from build123d import *

# Parameters (mm, degrees)
SKETCH1_W           = 20
SKETCH1_H           = 20
BOSS_EXTRUDE1_DEPTH = 6
BOSS_EXTRUDE2_DEPTH = 26
SKETCH5_R           = 2
CUT_EXTRUDE1_DEPTH  = 32.176914536
CIRPATTERN1_COUNT   = 2
CIRPATTERN1_ANGLE   = 90
BOSS_EXTRUDE3_DEPTH = 20
SKETCH6_R           = 2
CUT_EXTRUDE2_DEPTH  = 38.416573868
CIRPATTERN2_COUNT   = 2
CIRPATTERN2_ANGLE   = 90
FILLET1_R           = 1


with BuildPart() as part:
    # Sketch1 → Boss-Extrude1 (new body)
    with BuildSketch(Plane(origin=(0, 0, 0), x_dir=(1, 0, 0), z_dir=(0, 1, 0))):
        Rectangle(SKETCH1_W, SKETCH1_H)
    extrude(amount=BOSS_EXTRUDE1_DEPTH)

    # Sketch2 → Boss-Extrude2 (add)
    with BuildSketch(Plane(origin=(0, 0, 0), x_dir=(1, 0, 0), z_dir=(0, 1, 0))):
        Polygon((-3, 10), (3, 10), (3, 8.1), (5.3, 8.1), (5.3, 6.48), (2.8, 4), (-2.8, 4), (-5.3, 6.48), (-5.3, 8.1), (-3, 8.1), align=None)
    boss_extrude2 = extrude(amount=BOSS_EXTRUDE2_DEPTH)

    # Sketch5 → Cut-Extrude1 (cut, through all)
    with BuildSketch(Plane.XY.offset(-4)):
        with Locations((0, 18)):
            Circle(SKETCH5_R)
    cut_extrude1 = extrude(amount=-CUT_EXTRUDE1_DEPTH, mode=Mode.SUBTRACT)

    # CirPattern1: Boss-Extrude2, Cut-Extrude1 ×2 about axis
    cirpattern1_axis = Axis((0, 0, 0), (0, 1, 0))
    add([boss_extrude2.rotate(cirpattern1_axis, i * CIRPATTERN1_ANGLE / (CIRPATTERN1_COUNT - 1)) for i in range(1, CIRPATTERN1_COUNT)])
    add([cut_extrude1.rotate(cirpattern1_axis, i * CIRPATTERN1_ANGLE / (CIRPATTERN1_COUNT - 1)) for i in range(1, CIRPATTERN1_COUNT)], mode=Mode.SUBTRACT)

    # Sketch4 → Boss-Extrude3 (add)
    with BuildSketch(Plane(origin=(10, 6.045130441, 0.430052004), x_dir=(0, 0, 1), z_dir=(1, 0, 0))):
        Polygon((-3.430052004, 6.045130441), (2.569947996, 6.045130441), (2.569947996, 4.145130441), (4.869947996, 4.145130441), (4.869947996, 2.525130441), (2.369947996, 0.045130441), (-3.230052004, 0.045130441), (-5.730052004, 2.525130441), (-5.730052004, 4.145130441), (-3.430052004, 4.145130441), align=None)
    boss_extrude3 = extrude(amount=BOSS_EXTRUDE3_DEPTH)

    # Sketch6 → Cut-Extrude2 (cut, through all)
    with BuildSketch(Plane(origin=(0, 6, 0), x_dir=(1, 0, 0), z_dir=(0, 1, 0))):
        with Locations(Location((22, 0, 0), (0, 0, 270))):
            Circle(SKETCH6_R)
    cut_extrude2 = extrude(amount=-CUT_EXTRUDE2_DEPTH, mode=Mode.SUBTRACT)

    # CirPattern2: Boss-Extrude3, Cut-Extrude2 ×2 about axis
    cirpattern2_axis = Axis((0, 0, 0), (0, -1, 0))
    add([boss_extrude3.rotate(cirpattern2_axis, i * CIRPATTERN2_ANGLE / (CIRPATTERN2_COUNT - 1)) for i in range(1, CIRPATTERN2_COUNT)])
    add([cut_extrude2.rotate(cirpattern2_axis, i * CIRPATTERN2_ANGLE / (CIRPATTERN2_COUNT - 1)) for i in range(1, CIRPATTERN2_COUNT)], mode=Mode.SUBTRACT)

    # Fillet1
    fillet1_edges = [part.edges().sort_by_distance(p)[0] for p in [
        (-10, 0, 0),
        (0, 0, -10),
        (10, 3, -10),
        (10, 3, 10),
        (-10, 3, 10),
        (-10, 3, -10),
    ]]
    fillet(fillet1_edges, radius=FILLET1_R)


solid = part.part
Can you work these out from the model? Positions are in its coordinate system, mm. A direction names the side the tool comes from. Give positions to 0.01 mm unless a question says otherwise; leave off trailing zeros. Order: outer loops, then holes, each group sorted by start corner. A loop starts at its lowest first (then second) coordinate and runs counter-clockwise, first axis right, second up. Notation, with made-up numbers: M -28.75,-34 L 0.25,-34 A16 cw 0.25,-25 Z; hole C 43.25,7 d6. An arc over 180 degrees is marked long. One line per item, written item: value.
Item 1: If we section it at D-D on x = 0: Write out the boundary of the cut face in (y, z), and give its area (3 significant figures).
Verdict:
outline: M 0,-9 A1 ccw 1,-10 L 16,-10 L 16,-4 L 6,-4 L 6,20 L 0,20 Z; M 0,24 L 6,24 L 6,30 L 0,30 Z; M 20,-10 L 26,-10 L 26,-4 L 20,-4 Z
area: 312 mm2
Item 2: If we section it at B-B on x = 22: Write out the boundary of the cut face in (y, z), and give its area (3 significant figures).
Verdict:
outline: M 0,-3 L 1.9,-3 L 1.9,-5.3 L 3.52,-5.3 L 6,-2.8 L 6,-2 L 0,-2 Z; M 0,2 L 6,2 L 6,2.8 L 3.52,5.3 L 1.9,5.3 L 1.9,3 L 0,3 Z
area: 24.7 mm2
Item 3: For pin 1 (0.6 mm diameter, centred on y = 13, z = -9.5, fed in from +X); pin 2 (1 mm diameter, centred on x = -2.5, z = 26, fed in from +Y); pin 3 (1.8 mm diameter, centred on x = -7.5, y = 14.5, fed in from -Z), each with a flat end and sliding along its axis, tell me the tip position at first contact or that it passes through.
Verdict:
pin 1: x = 3
pin 2: y = 6
pin 3: z = -5.3
Item 4: If we mould it in two halves opening along X, with no side actions, what happens to faces 1 (the face through (-5.22, 15.86, 4.03)), 2 (the face through (-5.3, 3, 20)), 3 (the face through (20.8, 3, -1.6)), 4 (the face through (-5.26, 15.86, -4.07))? For each: pulls with the +X half, pulls with the -X half, needs draft (parallel to the pull), parting line crosses it, or undercut.
Verdict:
face 1: pulls with the +X half
face 2: pulls with the -X half
face 3: undercut
face 4: undercut
Item 5: If we section it at A-A on z = 22: Write out the boundary of the cut face in (x, y).
Verdict:
outline: M -5.3,1.9 L -3,1.9 L -3,0 L -2,0 L -2,6 L -2.8,6 L -5.3,3.52 Z; M 2,0 L 3,0 L 3,1.9 L 5.3,1.9 L 5.3,3.52 L 2.8,6 L 2,6 Z
Item 6: Please list where these lines run through material, in increasing order: line 1 (Y direction, x = 0, z = -5.5); line 2 (X direction, y = 1.55, z = 0); line 3 (X direction, y = 1, z = 17.5).
Verdict:
line 1: 0 to 16, 20 to 26
line 2: -10 to 20, 24 to 30
line 3: -3 to 3
Item 7: If we section it at C-C on y = 14.25: Write out the boundary of the cut face in (x, z).
Verdict:
outline: M -10,-3 L -8.1,-3 L -8.1,-5.3 L -6.48,-5.3 L -4,-2.8 L -4,2.8 L -6.48,5.3 L -8.1,5.3 L -8.1,3 L -10,3 Z; M -5.3,-8.1 L -3,-8.1 L -3,-10 L 3,-10 L 3,-8.1 L 5.3,-8.1 L 5.3,-6.48 L 2.8,-4 L -2.8,-4 L -5.3,-6.48 Z
Item 8: For faces 5 (the face through (-4.03, 15.86, -5.22)), 6 (the face through (-7, 3, 10)), 7 (the face through (5.3, 16, -7)), 8 (the face through (-4, 16, -1)), 9 (the face through (-4, 16, -8.1)), which set-ups out of +Z, -Z, +X, -X, +Y, -Y let a thin tool reach every point of the face, with its end or its side?
Verdict:
face 5: +Y
face 6: +Z, -X
face 7: +Z, -Z, +X, +Y
face 8: +Z, +X, +Y
face 9: -Z, -X, +Y
